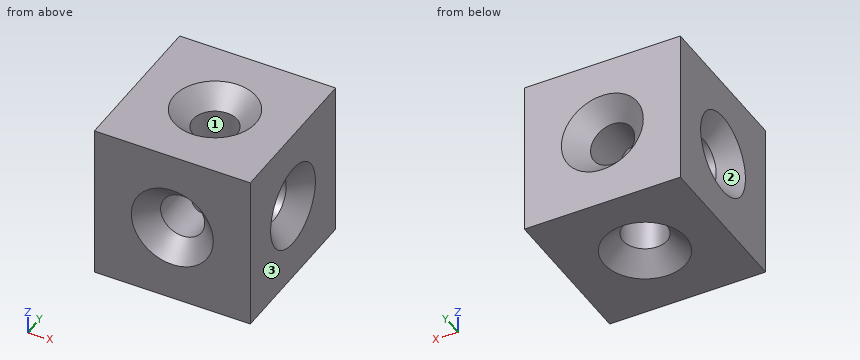
from build123d import *

# Parameters (mm, degrees)
SKETCH1_W                                       = 12
SKETCH1_H                                       = 12
BOSS_EXTRUDE1_DEPTH                             = 6
CSK_FOR_M3_FLAT_HEAD_MACHINE_SCREW1_D           = 3.4
CSK_FOR_M3_FLAT_HEAD_MACHINE_SCREW1_DEPTH       = 6
CSK_FOR_M3_FLAT_HEAD_MACHINE_SCREW1_CSINK_D     = 6.3
CSK_FOR_M3_FLAT_HEAD_MACHINE_SCREW1_CSINK_ANGLE = 90
CSK_FOR_M3_FLAT_HEAD_MACHINE_SCREW1_TIP         = 1.021463052
CSK_FOR_M3_FLAT_HEAD_MACHINE_SCREW2_D           = 3.4
CSK_FOR_M3_FLAT_HEAD_MACHINE_SCREW2_DEPTH       = 6
CSK_FOR_M3_FLAT_HEAD_MACHINE_SCREW2_CSINK_D     = 6.3
CSK_FOR_M3_FLAT_HEAD_MACHINE_SCREW2_CSINK_ANGLE = 90
CSK_FOR_M3_FLAT_HEAD_MACHINE_SCREW2_TIP         = 1.021463052
CSK_FOR_M3_FLAT_HEAD_MACHINE_SCREW3_D           = 3.4
CSK_FOR_M3_FLAT_HEAD_MACHINE_SCREW3_DEPTH       = 6
CSK_FOR_M3_FLAT_HEAD_MACHINE_SCREW3_CSINK_D     = 6.3
CSK_FOR_M3_FLAT_HEAD_MACHINE_SCREW3_CSINK_ANGLE = 90
CSK_FOR_M3_FLAT_HEAD_MACHINE_SCREW3_TIP         = 1.021463052
CSK_FOR_M3_FLAT_HEAD_MACHINE_SCREW7_D           = 3.4
CSK_FOR_M3_FLAT_HEAD_MACHINE_SCREW7_DEPTH       = 6
CSK_FOR_M3_FLAT_HEAD_MACHINE_SCREW7_CSINK_D     = 6.3
CSK_FOR_M3_FLAT_HEAD_MACHINE_SCREW7_CSINK_ANGLE = 90
CSK_FOR_M3_FLAT_HEAD_MACHINE_SCREW7_TIP         = 1.021463052
CSK_FOR_M3_FLAT_HEAD_MACHINE_SCREW8_D           = 3.4
CSK_FOR_M3_FLAT_HEAD_MACHINE_SCREW8_DEPTH       = 6
CSK_FOR_M3_FLAT_HEAD_MACHINE_SCREW8_CSINK_D     = 6.3
CSK_FOR_M3_FLAT_HEAD_MACHINE_SCREW8_CSINK_ANGLE = 90
CSK_FOR_M3_FLAT_HEAD_MACHINE_SCREW8_TIP         = 1.021463052
CSK_FOR_M3_FLAT_HEAD_MACHINE_SCREW9_D           = 3.4
CSK_FOR_M3_FLAT_HEAD_MACHINE_SCREW9_DEPTH       = 6
CSK_FOR_M3_FLAT_HEAD_MACHINE_SCREW9_CSINK_D     = 6.3
CSK_FOR_M3_FLAT_HEAD_MACHINE_SCREW9_CSINK_ANGLE = 90
CSK_FOR_M3_FLAT_HEAD_MACHINE_SCREW9_TIP         = 1.021463052


with BuildPart() as part:
    # Sketch1 → Boss-Extrude1 (new, symmetric)
    with BuildSketch(Plane.XY):
        Rectangle(SKETCH1_W, SKETCH1_H)
    extrude(amount=BOSS_EXTRUDE1_DEPTH, both=True)

    # CSK for M3 Flat Head Machine Screw1
    with Locations(Plane.XY.offset(6)):
        with Locations((0, 0)):
            CounterSinkHole(CSK_FOR_M3_FLAT_HEAD_MACHINE_SCREW1_D / 2, CSK_FOR_M3_FLAT_HEAD_MACHINE_SCREW1_CSINK_D / 2, depth=CSK_FOR_M3_FLAT_HEAD_MACHINE_SCREW1_DEPTH, counter_sink_angle=CSK_FOR_M3_FLAT_HEAD_MACHINE_SCREW1_CSINK_ANGLE)
            with Locations((0, 0, -(CSK_FOR_M3_FLAT_HEAD_MACHINE_SCREW1_DEPTH + CSK_FOR_M3_FLAT_HEAD_MACHINE_SCREW1_TIP / 2))):  # 118° drill point
                Cone(0, CSK_FOR_M3_FLAT_HEAD_MACHINE_SCREW1_D / 2, CSK_FOR_M3_FLAT_HEAD_MACHINE_SCREW1_TIP, mode=Mode.SUBTRACT)

    # CSK for M3 Flat Head Machine Screw2
    with Locations(Plane(origin=(6, 0, 0), x_dir=(0, 0, -1), z_dir=(1, 0, 0))):
        with Locations((0, 0)):
            CounterSinkHole(CSK_FOR_M3_FLAT_HEAD_MACHINE_SCREW2_D / 2, CSK_FOR_M3_FLAT_HEAD_MACHINE_SCREW2_CSINK_D / 2, depth=CSK_FOR_M3_FLAT_HEAD_MACHINE_SCREW2_DEPTH, counter_sink_angle=CSK_FOR_M3_FLAT_HEAD_MACHINE_SCREW2_CSINK_ANGLE)
            with Locations((0, 0, -(CSK_FOR_M3_FLAT_HEAD_MACHINE_SCREW2_DEPTH + CSK_FOR_M3_FLAT_HEAD_MACHINE_SCREW2_TIP / 2))):  # 118° drill point
                Cone(0, CSK_FOR_M3_FLAT_HEAD_MACHINE_SCREW2_D / 2, CSK_FOR_M3_FLAT_HEAD_MACHINE_SCREW2_TIP, mode=Mode.SUBTRACT)

    # CSK for M3 Flat Head Machine Screw3
    with Locations(Plane(origin=(0, 0, -6), x_dir=(-1, 0, 0), z_dir=(0, 0, -1))):
        with Locations((0, 0)):
            CounterSinkHole(CSK_FOR_M3_FLAT_HEAD_MACHINE_SCREW3_D / 2, CSK_FOR_M3_FLAT_HEAD_MACHINE_SCREW3_CSINK_D / 2, depth=CSK_FOR_M3_FLAT_HEAD_MACHINE_SCREW3_DEPTH, counter_sink_angle=CSK_FOR_M3_FLAT_HEAD_MACHINE_SCREW3_CSINK_ANGLE)
            with Locations((0, 0, -(CSK_FOR_M3_FLAT_HEAD_MACHINE_SCREW3_DEPTH + CSK_FOR_M3_FLAT_HEAD_MACHINE_SCREW3_TIP / 2))):  # 118° drill point
                Cone(0, CSK_FOR_M3_FLAT_HEAD_MACHINE_SCREW3_D / 2, CSK_FOR_M3_FLAT_HEAD_MACHINE_SCREW3_TIP, mode=Mode.SUBTRACT)

    # CSK for M3 Flat Head Machine Screw7
    with Locations(Plane.ZY.offset(6)):
        with Locations((0, 0)):
            CounterSinkHole(CSK_FOR_M3_FLAT_HEAD_MACHINE_SCREW7_D / 2, CSK_FOR_M3_FLAT_HEAD_MACHINE_SCREW7_CSINK_D / 2, depth=CSK_FOR_M3_FLAT_HEAD_MACHINE_SCREW7_DEPTH, counter_sink_angle=CSK_FOR_M3_FLAT_HEAD_MACHINE_SCREW7_CSINK_ANGLE)
            with Locations((0, 0, -(CSK_FOR_M3_FLAT_HEAD_MACHINE_SCREW7_DEPTH + CSK_FOR_M3_FLAT_HEAD_MACHINE_SCREW7_TIP / 2))):  # 118° drill point
                Cone(0, CSK_FOR_M3_FLAT_HEAD_MACHINE_SCREW7_D / 2, CSK_FOR_M3_FLAT_HEAD_MACHINE_SCREW7_TIP, mode=Mode.SUBTRACT)

    # CSK for M3 Flat Head Machine Screw8
    with Locations(Plane(origin=(0, 6, 0), x_dir=(1, 0, 0), z_dir=(0, 1, 0))):
        with Locations((0, 0)):
            CounterSinkHole(CSK_FOR_M3_FLAT_HEAD_MACHINE_SCREW8_D / 2, CSK_FOR_M3_FLAT_HEAD_MACHINE_SCREW8_CSINK_D / 2, depth=CSK_FOR_M3_FLAT_HEAD_MACHINE_SCREW8_DEPTH, counter_sink_angle=CSK_FOR_M3_FLAT_HEAD_MACHINE_SCREW8_CSINK_ANGLE)
            with Locations((0, 0, -(CSK_FOR_M3_FLAT_HEAD_MACHINE_SCREW8_DEPTH + CSK_FOR_M3_FLAT_HEAD_MACHINE_SCREW8_TIP / 2))):  # 118° drill point
                Cone(0, CSK_FOR_M3_FLAT_HEAD_MACHINE_SCREW8_D / 2, CSK_FOR_M3_FLAT_HEAD_MACHINE_SCREW8_TIP, mode=Mode.SUBTRACT)

    # CSK for M3 Flat Head Machine Screw9
    with Locations(Plane(origin=(0, -6, 0), x_dir=(-1, 0, 0), z_dir=(0, -1, 0))):
        with Locations((0, 0)):
            CounterSinkHole(CSK_FOR_M3_FLAT_HEAD_MACHINE_SCREW9_D / 2, CSK_FOR_M3_FLAT_HEAD_MACHINE_SCREW9_CSINK_D / 2, depth=CSK_FOR_M3_FLAT_HEAD_MACHINE_SCREW9_DEPTH, counter_sink_angle=CSK_FOR_M3_FLAT_HEAD_MACHINE_SCREW9_CSINK_ANGLE)
            with Locations((0, 0, -(CSK_FOR_M3_FLAT_HEAD_MACHINE_SCREW9_DEPTH + CSK_FOR_M3_FLAT_HEAD_MACHINE_SCREW9_TIP / 2))):  # 118° drill point
                Cone(0, CSK_FOR_M3_FLAT_HEAD_MACHINE_SCREW9_D / 2, CSK_FOR_M3_FLAT_HEAD_MACHINE_SCREW9_TIP, mode=Mode.SUBTRACT)


solid = part.part
Work out the finished part from the listing and answer in its coordinate system (mm). Face numbers are marked on the shaded views. Give positions to 0.01 mm unless a question says otherwise; leave off trailing zeros. Order: outer loops, then holes, each group sorted by start corner. A loop starts at its lowest first (then second) coordinate and runs counter-clockwise, first axis right, second up. Notation, with made-up numbers: (75.25, 29.25) -> (79.25, 29.25) arc R15 cw to (79.25, 41.25) -> close; hole circle Ø2 at (84.25, 31). An arc over 180 degrees is marked (long way). Answer as a JSON object with one key per item and string values. Group by question number.
1. Section A-A on y = 0 is taken. Determine the outline of the cut face in (x, z).
2. Flat-ended cylindrical pins translate along their axes: pin 1 Ø4 at (x, z) = (0, 0) entering from -Y; pin 2 Ø4.5 at (x, y) = (0, 0) entering from +Z. Find the tip coordinate at first contact, or state that the pin passes through.
3. Section C-C on x = 3.75 is taken. Determine the outline of the cut face in (y, z), plus the area to 3 significant figures.
4. Consider line 1 along X through (y, z) = (0, -3.3). Determine where the line is inside the solid, lowest interval first. Write a range as [from, to].
5. The mould has two halves that part along X. Classify the marked faces 1, 2 and 3: released by +X, released by -X, zero draft, split by the parting line, or undercut.
Result sheet:
{
 "1": {"outline": "(-6, -6) -> (-3.15, -6) -> (-1.7, -4.55) -> (-1.7, -1.7) -> (-4.55, -1.7) -> (-6, -3.15) -> close; (-6, 3.15) -> (-4.55, 1.7) -> (-1.7, 1.7) -> (-1.7, 4.55) -> (-3.15, 6) -> (-6, 6) -> close; (1.7, -4.55) -> (3.15, -6) -> (6, -6) -> (6, -3.15) -> (4.55, -1.7) -> (1.7, -1.7) -> close; (1.7, 1.7) -> (4.55, 1.7) -> (6, 3.15) -> (6, 6) -> (3.15, 6) -> (1.7, 4.55) -> close"},
 "2": {"pin 1": "stops at y = -4.85", "pin 2": "stops at z = 5.1"},
 "3": {"outline": "(-6, -6) -> (6, -6) -> (6, 6) -> (-6, 6) -> close; hole circle Ø3.4 at (0, 0)", "area": "135 mm^2"},
 "4": {"line 1": "x = [-6, -1.7], [1.7, 6]"},
 "5": {"face 1": "undercut", "face 2": "released by -X", "face 3": "released by +X"}
}
